```python
from build123d import *

# Parameters (mm, degrees)
F0_W     = 1905
F0_H     = 50.8
F1_DEPTH = 19.05
F2_W     = 50.8
F2_H     = 19.05
F3_DEPTH = 558.8
F4_W     = 50.8
F4_H     = 19.05
F5_DEPTH = 1854.2
F6_W     = 83.633751
F6_H     = 19.05
F6_W_2   = 92.737854
F7_DEPTH = 558.8


with BuildPart() as f1:
    # F0 (on Top) → F1 (new body)
    with BuildSketch(Plane.XY):
        with Locations((12.134612, 25.4)):
            Rectangle(F0_W, F0_H)
    extrude(amount=F1_DEPTH)

    # F2 (on face) → F3 (join)
    with BuildSketch(Plane.XZ):
        with Locations((-914.965388, 9.525)):
            Rectangle(F2_W, F2_H)
        with Locations((939.234612, 9.525)):
            Rectangle(F2_W, F2_H)
    extrude(amount=F3_DEPTH)

    # F4 (on face) → F5 (join)
    with BuildSketch(Plane.YZ.offset(-889.565388)):
        with Locations((-533.4, 9.525)):
            Rectangle(F4_W, F4_H)
    extrude(amount=F5_DEPTH)

    # F6 (on face) → F7 (join)
    with BuildSketch(Plane.XZ):
        with Locations((462.054446, 9.525)):
            Rectangle(F6_W, F6_H)
        with Locations((-477.944821, 9.525)):
            Rectangle(F6_W_2, F6_H)
    extrude(amount=F7_DEPTH)


solid = f1.part
```
CAD build for the part. Positions are in the model's coordinates, mm. Give positions to 0.01 mm unless a question says otherwise; leave off trailing zeros. Order: outer loops, then holes, each group sorted by start corner. A loop starts at its lowest first (then second) coordinate and runs counter-clockwise, first axis right, second up. Notation, with made-up numbers: M -28,6 L 16,6 A28 cw 16,30 Z; hole C 82.25,50 d6. An arc over 180 degrees is marked long. Put each result on its own line as item: value. Start each with the question number.
(1) Saw through at A-A, the plane x = -210.5. Write the cut outline in (y, z), then the cut area to 3 significant figures.
(2) Saw through at C-C, the plane z = 12.25. Write the cut outline in (x, y), then the cut area to 3 significant figures.
(3) Saw through at B-B, the plane y = -375. Write the cut outline in (x, z), then the cut area to 3 significant figures.
(4) Drill centre lines: line 1 along X through (y, z) = (-221.5, 13.75); line 2 along Y through (x, z) = (166.5, 14.5). Where is each one in solid material? Low to high.
Check result:
1. outline: M -558.8,0 L -508,0 L -508,19.05 L -558.8,19.05 Z; M 0,0 L 50.8,0 L 50.8,19.05 L 0,19.05 Z
1. area: 1,940 mm2
2. outline: M -940.37,-558.8 L 964.63,-558.8 L 964.63,50.8 L -940.37,50.8 Z; hole M -889.57,-508 L -524.31,-508 L -524.31,0 L -889.57,0 Z; hole M -431.58,-508 L 420.24,-508 L 420.24,0 L -431.58,0 Z; hole M 503.87,-508 L 913.83,-508 L 913.83,0 L 503.87,0 Z
2. area: 335,000 mm2
3. outline: M -940.37,0 L -889.57,0 L -889.57,19.05 L -940.37,19.05 Z; M -524.31,0 L -431.58,0 L -431.58,19.05 L -524.31,19.05 Z; M 420.24,0 L 503.87,0 L 503.87,19.05 L 420.24,19.05 Z; M 913.83,0 L 964.63,0 L 964.63,19.05 L 913.83,19.05 Z
3. area: 5,300 mm2
4. line 1: x = -940.37 to -889.57, -524.31 to -431.58, 420.24 to 503.87, 913.83 to 964.63
4. line 2: y = -558.8 to -508, 0 to 50.8
